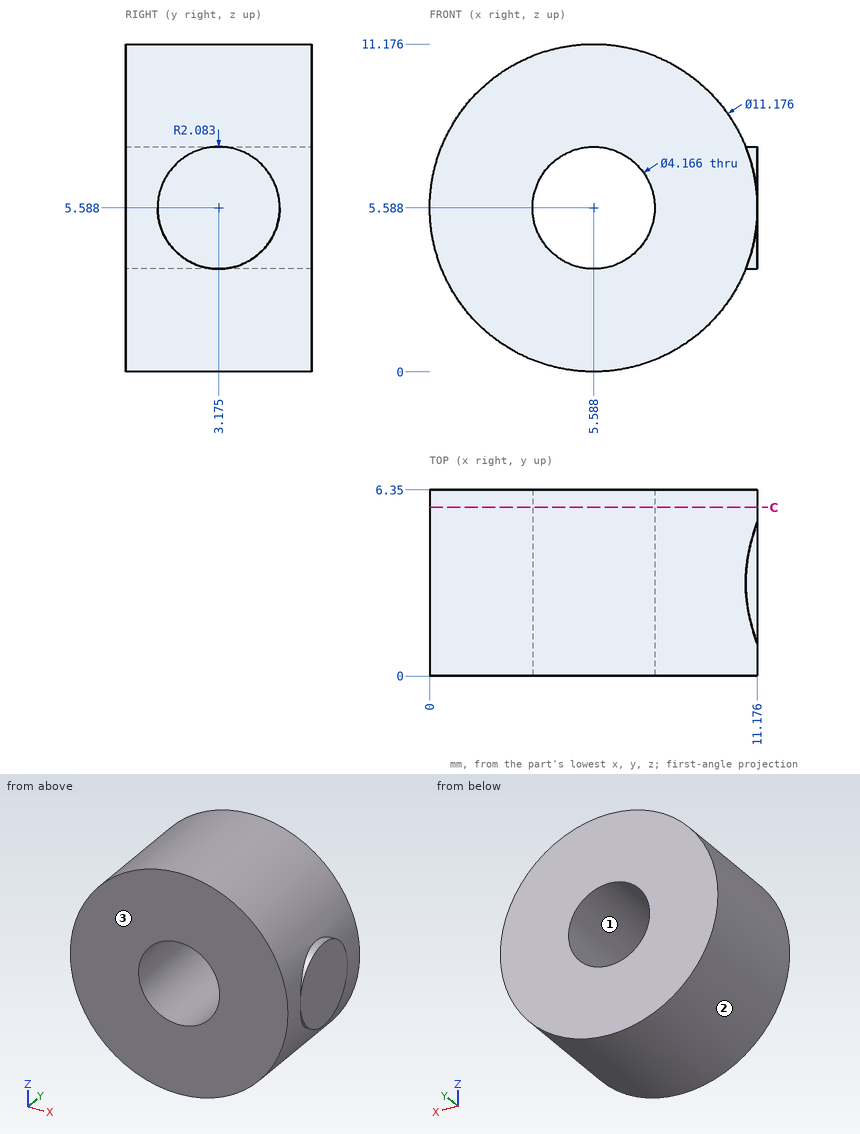
Could you check a few things on this drawing? It's one solid part, dimensions in mm from its lowest x, y, z. Coordinates: 2 decimals unless noted, no trailing zeros. Order: outer loops, then holes, each group sorted by start corner. A loop starts at its lowest first (then second) coordinate and runs counter-clockwise, first axis right, second up. Notation, with made-up numbers: (81.25, 20) - (110.25, 20) arc R13 ccw to (110.25, 39) - close; hole circle Ø2 at (85.25, -2). An arc over 180 degrees is marked (long way). Answer as a JSON object with one key per item and string values. Group by question number.
Q1. Imagine slicing it at C-C (y = 5.75). Please give me the cut outline in (x, z) (1 decimal).
Q2. We'd pull the mould along Z, two halves only. Please class the marked faces 1, 2 and 3: +Z half, -Z half, draft (parallel to the pull), parting line (faces both ways), or undercut.
Q3. I need wall thicknesses on line 1 (X direction, y = 4.75, z = 6.5) (1 decimal); line 2 (Z direction, x = 7.5, y = 2.75) (1 decimal); line 3 (Z direction, x = 5.75, y = 4.5) (1 decimal). Which ranges of each line are inside material? Lowest first, please. Write a range as from..to.
Determined:
{
 "1": {"outline": "circle Ø11.2 at (5.6, 5.6); hole circle Ø4.2 at (5.6, 5.6)"},
 "2": {"face 1": "undercut", "face 2": "parting line", "face 3": "draft"},
 "3": {"line 1": "x = 0.1..3.7, 7.5..11.2", "line 2": "z = 0.3..4.8, 6.4..10.8", "line 3": "z = 0..3.5, 7.7..11.2"}
}
